Can you work these out from the drawing? Everything is in mm from the part's minimum corner. A direction names the side the tool comes from. Coordinates: 2 decimals unless noted, no trailing zeros. Order: outer loops, then holes, each group sorted by start corner. A loop starts at its lowest first (then second) coordinate and runs counter-clockwise, first axis right, second up. Notation, with made-up numbers: (47.5, 51.5) - (60.5, 51.5) arc R6 cw to (60.5, 62.5) - close; hole circle Ø11 at (53.5, 11.25). An arc over 180 degrees is marked (long way). One line per item, written item: value.
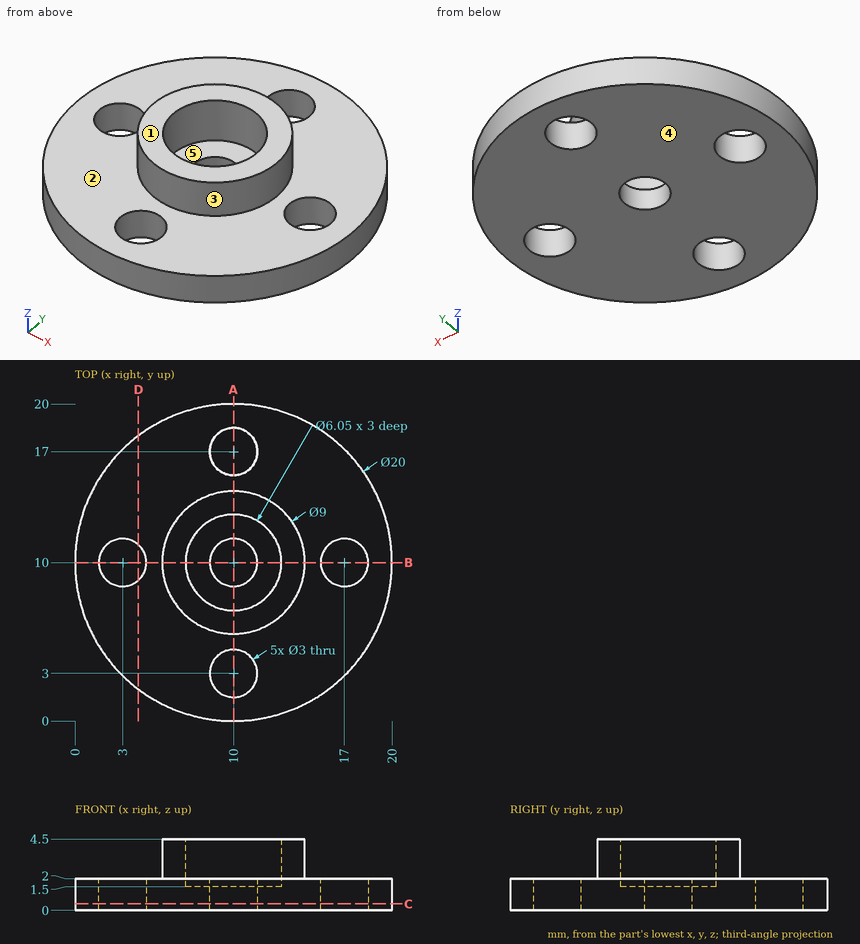
Item 1: I want a section at A-A on x = 10. Please give me the cut outline in (y, z) (3 decimals).
Conclusion:
outline: (0, 0) - (1.5, 0) - (1.5, 2) - (0, 2) - close; (4.5, 0) - (8.5, 0) - (8.5, 1.5) - (6.975, 1.5) - (6.975, 4.5) - (5.5, 4.5) - (5.5, 2) - (4.5, 2) - close; (11.5, 0) - (15.5, 0) - (15.5, 2) - (14.5, 2) - (14.5, 4.5) - (13.025, 4.5) - (13.025, 1.5) - (11.5, 1.5) - close; (18.5, 0) - (20, 0) - (20, 2) - (18.5, 2) - close
Item 2: Thinking about a two-plate mould opening in Y: for the marked faces 3, 4 and 5, which applies, pulls with the +Y half, pulls with the -Y half, needs draft (parallel to the pull), parting line crosses it, or undercut?
Conclusion:
face 3: parting line crosses it
face 4: needs draft
face 5: undercut
Item 3: If I drill on probe 1 along Y at (x, z) = (10, 0.55); probe 2 along Z at (x, y) = (16.75, 3.5); probe 3 along X at (y, z) = (10.5, 3.85), over which ranges is the centre line in solid material (lowest first)?
Conclusion:
probe 1: 0 to 1.5, 4.5 to 8.5, 11.5 to 15.5, 18.5 to 20
probe 2: 0 to 2
probe 3: 5.53 to 7.02, 12.98 to 14.47
Item 4: I want a section at C-C on z = 0.4. Please give me the cut outline in (x, y).
Conclusion:
outline: circle Ø20 at (10, 10); hole circle Ø3 at (3, 10); hole circle Ø3 at (10, 3); hole circle Ø3 at (10, 10); hole circle Ø3 at (10, 17); hole circle Ø3 at (17, 10)
Item 5: I want a section at D-D on x = 4. Please give me the cut outline in (y, z), then the cut area to 3 significant figures.
Conclusion:
outline: (2, 0) - (8.88, 0) - (8.88, 2) - (2, 2) - close; (11.12, 0) - (18, 0) - (18, 2) - (11.12, 2) - close
area: 27.5 mm²
Item 6: For the marked faces 1 and 2, which set-ups out of +Z, -Z, +X, -X, +Y, -Y let a thin tool reach every point of the face, with its end or its side?
Conclusion:
face 1: +Z, +X, -X, +Y, -Y
face 2: +Z
Item 7: I'm going to push flat-ended pins straight in: pin 1 Ø9.5 at (x, y) = (10, 10) entering from +Z; pin 2 Ø2 at (x, z) = (6.5, 4) entering from -Y. Where does each tip first touch, or does it pass through?
Conclusion:
pin 1: z = 4.5
pin 2: y = 6.26
